Job drawing, mm, ordinate dimensions from the low corner. One solid piece. A direction names the side the tool comes from. Give positions to 0.01 mm unless a question says otherwise; leave off trailing zeros. Write each loop counter-clockwise with the first axis right and the second up, starting at its lowest first coordinate (ties: lowest second). Pieces come first, ordered by that corner, then holes. Notation, with made-up numbers: (81.25, 13) -> (133.25, 13) arc R22 cw to (133.25, 24) -> close; hole circle Ø9 at (41.25, 55.25). An arc over 180 degrees is marked (long way). Put each result on its own line as item: value. Start each with the question number.
Item 1: Slice it at A-A, the plane z = 10. List the corners of the cut face in (x, y).
Item 2: Tool access for the marked faces 1 and 2: list every direction of +Z, -Z, +X, -X, +Y, -Y with a clear straight run to the whole face (end or side of a thin tool).
Item 3: Drill centre lines: line 1 along X through (y, z) = (0.9, 6.35); line 2 along Z through (x, y) = (127, 1.35); line 3 along Y through (x, z) = (115, 4). Where is each one in solid material? Low to high.
Item 4: Flat gauge pins, fed straight in: pin 1 Ø2 at (y, z) = (3.5, 5.5) entering from +X; pin 2 Ø1 at (y, z) = (4.5, 1.5) entering from +X. Where does each tip first touch, or does it go through?
Item 5: Slice it at B-B, the plane y = 3.65. List the corners of the cut face in (x, z), plus the area to 3 significant figures.
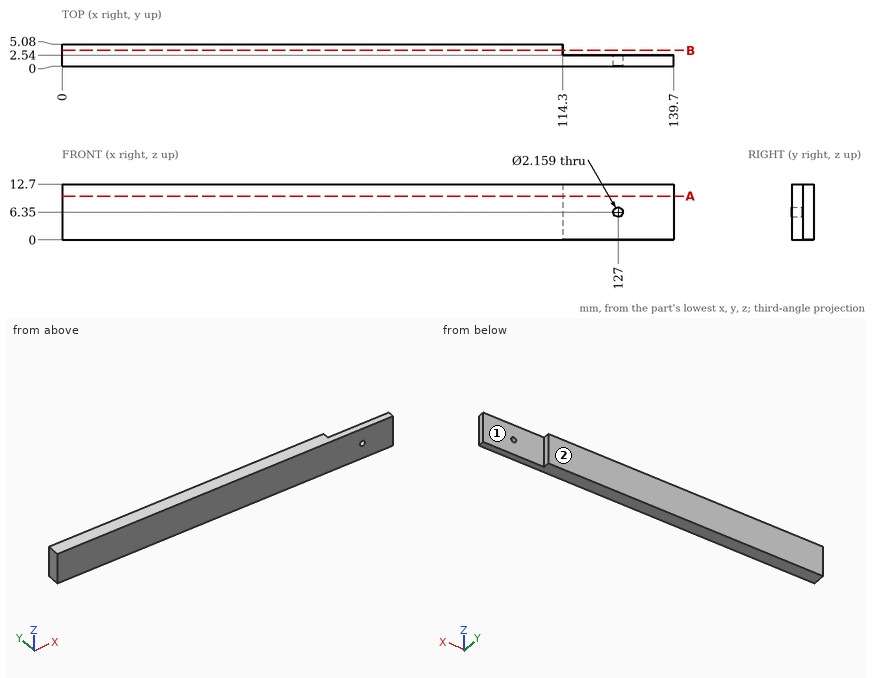
Values follow:
1. outline: (0, 0) -> (139.7, 0) -> (139.7, 2.54) -> (114.3, 2.54) -> (114.3, 5.08) -> (0, 5.08) -> close
2. face 1: +Z, -Z, +X, +Y
2. face 2: +Z, -Z, +X, -X, +Y
3. line 1: 0 to 125.92, 128.08 to 139.7
3. line 2: 0 to 5.27, 7.43 to 12.7
3. line 3: 0 to 2.54
4. pin 1: x = 139.7
4. pin 2: x = 114.3
5. outline: (0, 0) -> (114.3, 0) -> (114.3, 12.7) -> (0, 12.7) -> close
5. area: 1,450 mm2
